```python
from build123d import *

# Parameters (mm, degrees)
SKETCH_1_W          = 50
SKETCH_1_H          = 50
SKETCH_1_R          = 2
EXTRUDE_1_DEPTH     = 10
SKETCH_2_R          = 22
SKETCH_2_R_2        = 7.5
CUT_EXTRUDE_2_DEPTH = 9
CUT_EXTRUDE_3_DEPTH = 1


with BuildPart() as part:
    # 草图1 → 凸台-拉伸1 (new body)
    with BuildSketch(Plane(origin=(0, 0, 0), x_dir=(1, 0, 0), z_dir=(0, 1, 0))):
        with Locations((25, 25)):
            Rectangle(SKETCH_1_W, SKETCH_1_H)
        with Locations(Location((5, 45, 0), (0, 0, 270))):
            Circle(SKETCH_1_R, mode=Mode.SUBTRACT)
        with Locations(Location((45, 45, 0), (0, 0, 270))):
            Circle(SKETCH_1_R, mode=Mode.SUBTRACT)
        with Locations(Location((45, 5, 0), (0, 0, 270))):
            Circle(SKETCH_1_R, mode=Mode.SUBTRACT)
        with Locations(Location((5, 5, 0), (0, 0, 270))):
            Circle(SKETCH_1_R, mode=Mode.SUBTRACT)
    extrude(amount=EXTRUDE_1_DEPTH)

    # 草图2 → 切除-拉伸2 (cut)
    with BuildSketch(Plane(origin=(0, 10, 0), x_dir=(1, 0, 0), z_dir=(0, 1, 0))):
        with Locations(Location((25, 25, 0), (0, 0, 270))):
            Circle(SKETCH_2_R)
        with Locations(Location((25, 25, 0), (0, 0, 270))):
            Circle(SKETCH_2_R_2, mode=Mode.SUBTRACT)
    extrude(amount=-CUT_EXTRUDE_2_DEPTH, mode=Mode.SUBTRACT)

    # 草图3 → 切除-拉伸3 (cut)
    with BuildSketch(Plane(origin=(0, 1, 0), x_dir=(1, 0, 0), z_dir=(0, 1, 0))):
        with BuildLine():
            Line((24.216036525, 32.458914215), (22.700373808, 46.879481698))
            ThreePointArc((22.700373808, 46.879481698), (26.151391037, 3.030150235), (25, 47))
            Line((25, 47), (25, 32.5))
            ThreePointArc((25, 32.5), (25.392519672, 17.510278489), (24.216036525, 32.458914215))
        make_face()
    extrude(amount=-CUT_EXTRUDE_3_DEPTH, mode=Mode.SUBTRACT)


solid = part.part
```
Input: part model. Units: mm. Frame: model coordinates. A direction names the side the tool comes from. Give positions to 0.01 mm unless a question says otherwise; leave off trailing zeros. Write each loop counter-clockwise with the first axis right and the second up, starting at its lowest first coordinate (ties: lowest second). Pieces come first, ordered by that corner, then holes. Notation, with made-up numbers: (75.5, 6.5) - (128.5, 6.5) arc R27 ccw to (128.5, 25.5) - close; hole circle Ø10 at (76.25, 84.5). An arc over 180 degrees is marked (long way). Write item = value, one per line. Start each with the question number.
1) Cut plane D-D (z = -25). Return loops of the section in (x, y).
2) Cut plane C-C (x = 18.5). Return loops of the section in (y, z).
3) Cut plane B-B (z = -45). Return loops of the section in (x, y), and give its area (3 significant figures).
4) Reachability of faces 1 (the face through (24, 1, -41)), 2 (the face through (23.47, 0.51, -39.57)), 3 (the face through (25, 10, -25)) from +Z, -Z, +X, -X, +Y, -Y: full face, straight path, thin tool, end or side. Return the list, or none.
5) Cut plane A-A (y = 7). Return loops of the section in (x, z).
6) Draft query along Z for faces 4 (the face through (5, 5, -47)), 5 (the face through (6.352, 4.93, -6.474)), 6 (the face through (50, 5, -25)), 7 (the face through (25, 5, 0)). Return one class per face: pulls with the +Z half, pulls with the -Z half, needs draft (parallel to the pull), parting line crosses it, or undercut.
7) Material intervals for L1, parallel to X at y = 0.25, z = -25; L2, parallel to Z at x = 31.5, y = 9.5; L3, parallel to X at y = 7, z = -45, sorted ascending. Write a range as [from, to].
8) Pin query (flat end, axial travel): pin 1 (1.8 mm diameter, centred on x = 23.5, z = -40, fed in from +Y); pin 2 (3.5 mm diameter, centred on x = 45, z = -5, fed in from +Y). Return the tip coordinate at first contact, or that it passes through.
Answers follow:
q1.outline = (0, 0) - (3, 0) - (3, 10) - (0, 10) - close; (17.5, 0) - (32.5, 0) - (32.5, 10) - (17.5, 10) - close; (47, 0) - (50, 0) - (50, 10) - (47, 10) - close
q2.outline = (0, -50) - (10, -50) - (10, -46.02) - (0, -46.02) - close; (0, -28.74) - (10, -28.74) - (10, -21.26) - (0, -21.26) - close; (0, -3.98) - (10, -3.98) - (10, 0) - (0, 0) - close
q3.outline = (0, 0) - (3, 0) - (3, 10) - (0, 10) - close; (7, 0) - (15.83, 0) - (15.83, 10) - (7, 10) - close; (22.9, 0) - (25, 0) - (25, 1) - (22.9, 1) - close; (34.17, 0) - (43, 0) - (43, 10) - (34.17, 10) - close; (47, 0) - (50, 0) - (50, 10) - (47, 10) - close
q3.area = 239 mm^2
q4.face_1 = +Y
q4.face_2 = +Y, -Y
q4.face_3 = +Z, -Z, +X, -X, +Y
q5.outline = (0, -50) - (50, -50) - (50, 0) - (0, 0) - close; circle Ø15 at (25, -25); hole circle Ø4 at (5, -45); hole circle Ø44 at (25, -25); hole circle Ø4 at (5, -5); hole circle Ø4 at (45, -45); hole circle Ø4 at (45, -5)
q6.face_4 = undercut
q6.face_5 = undercut
q6.face_6 = needs draft
q6.face_7 = pulls with the +Z half
q7.L1 = [0, 3], [17.5, 32.5], [47, 50]
q7.L2 = [-50, -46.02], [-28.74, -21.26], [-3.98, 0]
q7.L3 = [0, 3], [7, 15.83], [34.17, 43], [47, 50]
q8.pin_1 = 1
q8.pin_2 = through
